Autodesk Fusion 360 part; units mm, degrees
sketch "Esquisse1" plane through (0, 0, 0) normal (0, 1, 0) x (1, 0, 0)
  line L0 (20.25, 5) -> (-20.25, 5)
  line L1 (-20.25, 5) -> (-20.25, -5)
  line L2 (-20.25, -5) -> (20.25, -5)
  line L3 (20.25, -5) -> (20.25, 5)
  line L4 (20.25, 5) -> (-20.25, -5) construction
  line L5 (-20.25, 5) -> (20.25, -5) construction
  dimension "d1" = 40.5
  dimension "d2" = 10
extrude "Extrusion1" add sketch "Esquisse1" along normal blind 4
sketch "Esquisse5" plane through (0, 0, 0) normal (0, 1, 0) x (1, 0, 0)
  line L0 (-10.25, 5) -> (-20.25, 5)
  line L1 (-20.25, 5) -> (-20.25, -5)
  line L2 (-20.25, -5) -> (-10.25, -5)
  line L3 (-10.25, -5) -> (-10.25, 5)
  line L4 (-10.25, 5) -> (-20.25, -5) construction
  line L5 (-20.25, 5) -> (-10.25, -5) construction
  circle A0 centre (-15.25, 0) radius 1.6
  line L6 (20.25, 5) -> (-20.25, 5)
  point P0 (-15.25, 0)
  dimension "d26" = 10
  dimension "d27" = 10
  dimension "d28" = 15.25
  dimension "d29" = 3.2
  dimension "d46" = 5
extrude "Extrusion7" add sketch "Esquisse5" along normal blind 12.5
extrude "Extrusion8" cut sketch "Esquisse5" along normal blind 4 contours A0
sketch "Esquisse6" plane through (0, 0, 0) normal (0, 1, 0) x (1, 0, 0)
  line L0 (20.25, -5) -> (20.25, 5)
  line L1 (10.25, 5) -> (20.25, -5) construction
  line L2 (10.25, 5) -> (10.25, -5)
  line L3 (20.25, 5) -> (10.25, 5)
  line L4 (10.25, -5) -> (20.25, -5)
  circle A0 centre (15.25, 0) radius 1.6
  line L5 (20.25, 5) -> (10.25, -5) construction
  line L6 (20.25, 5) -> (-20.25, 5)
  point P0 (15.25, 0)
  point P1 (28, 0)
  point P2 (28, 0)
  dimension "d34" = 10
  dimension "d35" = 10
  dimension "d37" = 3.2
  dimension "d38" = 15.25
  dimension "d47" = 5
extrude "Extrusion9" add sketch "Esquisse6" along normal blind 12.5
extrude "Extrusion10" cut sketch "Esquisse6" along normal blind 4 contours A0
chamfer "Chanfrein3" distance 2.1 angle 45 2 edges at (-16.7417, 0, 0.5786) (13.7583, 0, 0.5786)
sketch "Esquisse8" plane through (0, 4, 0) normal (0, 1, 0) x (-1, 0, 0)
  line L0 (-10.25, 5) -> (-10.25, -5)
  line L1 (-10.25, -5) -> (10.25, -5)
  line L2 (10.25, -5) -> (10.25, 5)
  line L3 (10.25, 5) -> (-10.25, 5)
  line L4 (8.25, -3) -> (-8.25, -3)
  line L5 (-8.25, -3) -> (-8.25, 3)
  line L6 (-8.25, 3) -> (8.25, 3)
  line L7 (8.25, 3) -> (8.25, -3)
  line L8 (8.25, -3) -> (-8.25, 3) construction
  line L9 (-8.25, -3) -> (8.25, 3) construction
  dimension "d52" = 16.5
  dimension "d53" = 6
extrude "Extrusion12" cut sketch "Esquisse8" against normal blind 2 contours L4 L5 L6 L7
fillet "Congé1" radius 1 2 edges at (-10.25, 4, 0) (10.25, 4, 0)
fillet "Congé2" radius 1 14 edges at (-10.25, 8.75, 5) (-9.9571, 4.2929, 5) (0, 4, 5) (9.9571, 4.2929, 5) (10.25, 8.75, 5) (10.25, 8.75, -5) (9.9571, 4.2929, -5) (0, 4, -5) (-9.9571, 4.2929, -5) (-10.25, 8.75, -5) (20.25, 6.25, 5) (-20.25, 6.25, -5) (20.25, 6.25, -5) (-20.25, 6.25, 5)
fillet "Congé3" radius 2 8 edges at (20.25, 0, 0) (19.9571, 0, -4.7071) (0, 0, -5) (-19.9571, 0, -4.7071) (-20.25, 0, 0) (-19.9571, 0, 4.7071) (0, 0, 5) (19.9571, 0, 4.7071)
fillet "Congé4" radius 1 6 edges at (0, 2, -3) (8.25, 2, 0) (-8.25, 2, 0) (0, 2, 3) (-8.25, 4, 0) (8.25, 4, 0)
equation "d1 = Linear Dimension-2"
equation "d2 = largeur_pont"
equation "d3 = epaisseur_pont"
equation "hauteur_pont = 8.5 mm"
equation "longueur_pile = vis_dia_tete + 3 mm"
equation "vis_dia_percage = 3.2 mm"
equation "epaisseur_pont = 4 mm"
equation "largeur_pont = vis_dia_tete + 3 mm"
equation "d26 = longueur_pile"
equation "d27 = largeur_pont"
equation "d28 = Linear Dimension-4"
equation "d29 = vis_dia_percage"
equation "d30 = epaisseur_pont + hauteur_pont"
equation "d32 = epaisseur_pont"
equation "d34 = longueur_pile"
equation "d35 = largeur_pont"
equation "d37 = vis_dia_percage"
equation "d38 = Linear Dimension-4"
equation "d39 = hauteur_pont + epaisseur_pont"
equation "d41 = epaisseur_pont"
equation "vis_dia_tete = 7 mm"
equation "d46 = largeur_pont / 2"
equation "d47 = largeur_pont / 2"
equation "d52 = Linear Dimension-2"
equation "d53 = largeur_pont - 4 mm"
equation "d54 = -epaisseur_pont + 2 mm"
equation "d58 = ( vis_dia_tete - vis_dia_percage ) / 2 + 0.2 mm"
CAD build for the part. Positions are in the model's coordinates, mm. A direction names the side the tool comes from. Round coordinates to 2 decimals unless told otherwise and drop trailing zeros. Loops run counter-clockwise (first coordinate to the right, second up) from the corner with the lowest first, then second, coordinate; pieces in that order, holes last. Notation, with made-up numbers: M 80,29 L 108,29 A8 cw 108,42 Z; hole C 21.5,-39 d11. An arc over 180 degrees is marked long. Return JSON: item names as keys, results as strings. Group by question number.
(1) Tool access for faces 4 (the flat face through (0.1, 3.5, 3)), 5 (the cylindrical face through (10.551, 8.698, 4.715)), 6 (the cylindrical face through (19.9, 0.87, 2.87)), 7 (the cylindrical face through (-18.12, 0.87, 4.65)), 8 (the cylindrical face through (-9.965, 4.301, 0.056)): list every direction of +Z, -Z, +X, -X, +Y, -Y with a clear straight run to the whole face (end or side of a thin tool).
(2) Saw through at A-A, the plane y = 5.75. List the corners of the cut face in (x, z), and give its area (3 significant figures).
(3) Drop flat-ended pins along their axis: P1, Ø1.1, axis at x = 4, y = 3.5, coming from the -Z side; P2, Ø3, axis at x = -0.5, y = 6, coming from the -Z side; P3, Ø4, axis at x = -15.25, z = 0, coming from the -Y side; P4, Ø2.5, axis at x = 4.5, z = -1.5, coming from the +Y side. Give the stop position or say it passes through.
(4) Wall check: probe 1 along X at (y, z) = (7.75, 0); probe 2 along Z at (x, y) = (15.25, 9); probe 3 along X at (y, z) = (2.5, 0.75). Give the ranges that are in metal, low to high. Write a range as [from, to].
(5) Mould opens along Z. For faces 1 (the cylindrical face through (-8.551, 3.715, -0.042)), 2 (the flat face through (10.25, 9, 0)), 3 (the cylindrical face through (-0.18, 0.6, -4.43)) say: +Z half, -Z half, draft (parallel to the pull), parting line (faces both ways), or undercut.
Answer list:
{
 "1": {"face 4": "+Y", "face 5": "+Z, +Y", "face 6": "+Z, +X, -Y", "face 7": "+Z, -X, -Y", "face 8": "+Z, -Z, +Y"},
 "2": {"outline": "M -20.25,-4 A1 ccw -19.25,-5 L -11.25,-5 A1 ccw -10.25,-4 L -10.25,4 A1 ccw -11.25,5 L -19.25,5 A1 ccw -20.25,4 Z; M 10.25,-4 A1 ccw 11.25,-5 L 19.25,-5 A1 ccw 20.25,-4 L 20.25,4 A1 ccw 19.25,5 L 11.25,5 A1 ccw 10.25,4 Z; hole C -15.25,0 d3.2; hole C 15.25,0 d3.2", "area": "182 mm2"},
 "3": {"P1": "z = -5", "P2": "through", "P3": "y = 1.7", "P4": "y = 2.34"},
 "4": {"probe 1": "[-20.25, -16.85], [-13.65, -10.25], [10.25, 13.65], [16.85, 20.25]", "probe 2": "[-5, -1.6], [1.6, 5]", "probe 3": "[-20.25, -16.66], [-13.84, -8.12], [8.12, 13.84], [16.66, 20.25]"},
 "5": {"face 1": "undercut", "face 2": "draft", "face 3": "-Z half"}
}
